Here's how the part is built. I have some questions about the finished solid (model axes, mm). Coordinates: 2 decimals unless noted, no trailing zeros. Write each loop counter-clockwise with the first axis right and the second up, starting at its lowest first coordinate (ties: lowest second). Pieces come first, ordered by that corner, then holes. Notation, with made-up numbers: (-16, 72) -> (4, 72) arc R14 cw to (4, 77) -> close; hole circle Ø10 at (74, 48.5). An arc over 180 degrees is marked (long way). Answer in a Markdown table with one row per item. Add a question column.
from build123d import *

# Parameters (mm, degrees)
SKETCH_1_R      = 62.5
SKETCH_1_R_2    = 1.5
EXTRUDE_1_DEPTH = 1.5


with BuildPart() as part:
    # 草图1 → 凸台-拉伸1 (new body)
    with BuildSketch(Plane.XY):
        Circle(SKETCH_1_R)
        with Locations((0, -59)):
            Circle(SKETCH_1_R_2, mode=Mode.SUBTRACT)
        with Locations((-31.89780823, -49.633958437)):
            Circle(SKETCH_1_R_2, mode=Mode.SUBTRACT)
        with Locations((-53.668287726, -24.509485767)):
            Circle(SKETCH_1_R_2, mode=Mode.SUBTRACT)
        with Locations((-58.399465071, 8.396575458)):
            Circle(SKETCH_1_R_2, mode=Mode.SUBTRACT)
        with Locations((-44.589224887, 38.636783303)):
            Circle(SKETCH_1_R_2, mode=Mode.SUBTRACT)
        with Locations((-16.622220854, 56.610085443)):
            Circle(SKETCH_1_R_2, mode=Mode.SUBTRACT)
        with Locations((16.622220854, 56.610085443)):
            Circle(SKETCH_1_R_2, mode=Mode.SUBTRACT)
        with Locations((44.589224887, 38.636783303)):
            Circle(SKETCH_1_R_2, mode=Mode.SUBTRACT)
        with Locations((58.399465071, 8.396575458)):
            Circle(SKETCH_1_R_2, mode=Mode.SUBTRACT)
        with Locations((53.668287726, -24.509485767)):
            Circle(SKETCH_1_R_2, mode=Mode.SUBTRACT)
        with Locations((31.89780823, -49.633958437)):
            Circle(SKETCH_1_R_2, mode=Mode.SUBTRACT)
        with BuildLine():
            ThreePointArc((3.498460053, -58.896186441), (0, -55.5), (-3.498460053, -58.896186441))
            ThreePointArc((-3.498460053, -58.896186441), (-16.622220854, -56.610085443), (-28.898590503, -51.438035217))
            ThreePointArc((-28.898590503, -51.438035217), (-30.005565369, -46.689571072), (-34.784774262, -47.65521461))
            ThreePointArc((-34.784774262, -47.65521461), (-44.589224887, -38.636783303), (-52.120542762, -27.648671255))
            ThreePointArc((-52.120542762, -27.648671255), (-50.484575742, -23.055533222), (-55.027168419, -21.284048857))
            ThreePointArc((-55.027168419, -21.284048857), (-58.399465071, -8.396575458), (-58.794590961, 4.918950474))
            ThreePointArc((-58.794590961, 4.918950474), (-54.935090024, 7.898473524), (-57.798825407, 11.844652023))
            ThreePointArc((-57.798825407, 11.844652023), (-53.668287726, 24.509485767), (-46.801771952, 35.924840183))
            ThreePointArc((-46.801771952, 35.924840183), (-41.944101377, 36.344770734), (-42.219763715, 41.212759575))
            ThreePointArc((-42.219763715, 41.212759575), (-31.89780823, 49.633958437), (-19.949721034, 55.524846967))
            ThreePointArc((-19.949721034, 55.524846967), (-15.636156905, 53.251860036), (-13.236225354, 57.496107158))
            ThreePointArc((-13.236225354, 57.496107158), (0, 59), (13.236225354, 57.496107158))
            ThreePointArc((13.236225354, 57.496107158), (15.636156905, 53.251860036), (19.949721034, 55.524846967))
            ThreePointArc((19.949721034, 55.524846967), (31.89780823, 49.633958437), (42.219763715, 41.212759575))
            ThreePointArc((42.219763715, 41.212759575), (41.944101377, 36.344770734), (46.801771952, 35.924840183))
            ThreePointArc((46.801771952, 35.924840183), (53.668287726, 24.509485767), (57.798825407, 11.844652023))
            ThreePointArc((57.798825407, 11.844652023), (54.935090024, 7.898473524), (58.794590961, 4.918950474))
            ThreePointArc((58.794590961, 4.918950474), (58.399465071, -8.396575458), (55.027168419, -21.284048857))
            ThreePointArc((55.027168419, -21.284048857), (50.484575742, -23.055533222), (52.120542762, -27.648671255))
            ThreePointArc((52.120542762, -27.648671255), (44.589224887, -38.636783303), (34.784774262, -47.65521461))
            ThreePointArc((34.784774262, -47.65521461), (30.005565369, -46.689571072), (28.898590503, -51.438035217))
            ThreePointArc((28.898590503, -51.438035217), (16.622220854, -56.610085443), (3.498460053, -58.896186441))
        make_face(mode=Mode.SUBTRACT)
    extrude(amount=EXTRUDE_1_DEPTH)


solid = part.part
Q1. Imagine slicing it at D-D on x = -38.5. Please give me the cut outline in (y, z), plus the area to 3 significant figures.
Q2. Imagine slicing it at B-B on y = 0. Please give me the cut outline in (x, z).
Q3. Imagine slicing it at A-A on x = 0. Please give me the cut outline in (y, z), plus the area to 4 significant figures.
Q4. Imagine slicing it at C-C on z = 1.05. State how many separate pieces and enclosed holes the cut face has, plus the area to 3 significant figures.
Q5. I need wall thicknesses on line 1 (X direction, y = 39, z = 0.35); line 2 (Y direction, x = -50.5, z = 0.85); line 3 (Y direction, x = 45.5, z = 0.3). Which ranges of each line are inside material? Lowest first, please. Write a range as [from, to].
Q6. If we mould it in two halves opening along Y, with no side actions, what happens to faces 1 (the cylindrical face through (44.71, -38.5, 0.74)), 2 (the flat face through (14, 56, 0)), 3 (the cylindrical face through (-62.44, 2.75, 0.74))? For each: pulls with the +Y half, pulls with the -Y half, needs draft (parallel to the pull), parting line crosses it, or undercut.
Result sheet:
| question | item | result |
|---|---|---|
| 1 | outline | (-49.23, 0) -> (-44.71, 0) -> (-44.71, 1.5) -> (-49.23, 1.5) -> close; (44.71, 0) -> (49.23, 0) -> (49.23, 1.5) -> (44.71, 1.5) -> close |
| 1 | area | 13.6 mm^2 |
| 2 | outline | (-62.5, 0) -> (-59, 0) -> (-59, 1.5) -> (-62.5, 1.5) -> close; (59, 0) -> (62.5, 0) -> (62.5, 1.5) -> (59, 1.5) -> close |
| 3 | outline | (-62.5, 0) -> (-60.5, 0) -> (-60.5, 1.5) -> (-62.5, 1.5) -> close; (-57.5, 0) -> (-55.5, 0) -> (-55.5, 1.5) -> (-57.5, 1.5) -> close; (59, 0) -> (62.5, 0) -> (62.5, 1.5) -> (59, 1.5) -> close |
| 3 | area | 11.25 mm^2 |
| 4 | separate pieces | 1 |
| 4 | enclosed holes | 12 |
| 4 | area | 1,470 mm^2 |
| 5 | line 1 | x = [-48.84, -46.04], [-43.13, -41.11], [41.11, 43.13], [46.04, 48.84] |
| 5 | line 2 | y = [-36.82, -30.51], [-26, -23.02], [30.51, 36.82] |
| 5 | line 3 | y = [-42.85, -37.56], [35.26, 37.44], [39.83, 42.85] |
| 6 | face 1 | undercut |
| 6 | face 2 | needs draft |
| 6 | face 3 | parting line crosses it |
